```python
from build123d import *

# Parameters (mm, degrees)
SALIENTE_EXTRUIR1_DEPTH             = 30
SALIENTE_EXTRUIR1_2_DEPTH           = 30
SALIENTE_EXTRUIR1_3_DEPTH           = 30
SALIENTE_EXTRUIR1_4_DEPTH           = 30
SALIENTE_EXTRUIR3_REACH             = 48.233
CROQUIS3_W                          = 3.75
CROQUIS3_H                          = 31.257280714
SALIENTE_EXTRUIR3_DIRECTION_2_REACH = 48.233


with BuildPart() as part:
    # Croquis1 → Saliente-Extruir1 (new body)
    with BuildSketch(Plane.XY):
        Polygon((11.559312896, 31.017067239), (16.596862024, 31.017067239), (12.788445042, 0), (7.721401409, -0.240213475), align=None)
    extrude(amount=SALIENTE_EXTRUIR1_DEPTH)



with BuildPart() as body_2:
    # Croquis1 → Saliente-Extruir1 2 (new body)
    with BuildSketch(Plane.XY):
        Polygon((-7.529273594, 31.017067239), (-6.279253351, 20.836469336), (-6.279253351, 4.425451239), (-8.264345654, 20.592730649), (-9.544293245, 31.017067239), align=None)
    extrude(amount=SALIENTE_EXTRUIR1_2_DEPTH)


with BuildPart() as body_3:
    # Croquis1 → Saliente-Extruir1 3 (new body)
    with BuildSketch(Plane.XY):
        Polygon((-11.559312896, 31.017067239), (-7.721401409, -0.240213475), (-12.788445042, 0), (-16.596862024, 31.017067239), align=None)
    extrude(amount=SALIENTE_EXTRUIR1_3_DEPTH)


with BuildPart() as body_4:
    # Croquis1 → Saliente-Extruir1 4 (new body)
    with BuildSketch(Plane.XY):
        Polygon((7.529273594, 31.017067239), (6.279253351, 20.836469336), (6.279253351, 4.425451239), (8.264345654, 20.592730649), (9.544293245, 31.017067239), align=None)
    extrude(amount=SALIENTE_EXTRUIR1_4_DEPTH)


with BuildPart() as part_1:
    add(part.part)

    add(body_2.part)  # Saliente-Extruir3 merges body 2

    add(body_4.part)  # Saliente-Extruir3 merges body 4

    add(body_3.part)  # Saliente-Extruir3 merges body 3
    # Saliente-Extruir3: up to this plane
    saliente_extruir3_end = Plane(origin=(16.596862024, 31.017067239, 30), z_dir=(-0.992546151641322, 0.12186934340514874, 0))
    # Croquis3 → Saliente-Extruir3 (add, up to the surface)
    with BuildSketch(Plane(origin=(0, 0, 0), x_dir=(0, 0, -1), z_dir=(1, 0, 0)), mode=Mode.PRIVATE) as saliente_extruir3_sk1:
        with Locations((-28.125, 15.388426882)):
            Rectangle(CROQUIS3_W, CROQUIS3_H)
    saliente_extruir3_tool1 = split(extrude(saliente_extruir3_sk1.sketch, amount=SALIENTE_EXTRUIR3_REACH, mode=Mode.PRIVATE), bisect_by=saliente_extruir3_end, keep=Keep.BOTH, mode=Mode.PRIVATE)
    add(saliente_extruir3_tool1.solids().sort_by_distance((0, 15.388427, 28.125))[0])
    # Croquis3 → Saliente-Extruir3 (add, up to the surface)
    with BuildSketch(Plane(origin=(0, 0, 0), x_dir=(0, 0, -1), z_dir=(1, 0, 0)), mode=Mode.PRIVATE) as saliente_extruir3_sk2:
        with Locations((-1.875, 15.388426882)):
            Rectangle(CROQUIS3_W, CROQUIS3_H)
    saliente_extruir3_tool2 = split(extrude(saliente_extruir3_sk2.sketch, amount=SALIENTE_EXTRUIR3_REACH, mode=Mode.PRIVATE), bisect_by=saliente_extruir3_end, keep=Keep.BOTH, mode=Mode.PRIVATE)
    add(saliente_extruir3_tool2.solids().sort_by_distance((0, 15.388427, 1.875))[0])

    # Saliente-Extruir3 direction 2: up to this plane
    saliente_extruir3_direction_2_end = Plane(origin=(-16.596862024, 31.017067239, 30), z_dir=(0.992546151641322, 0.12186934340514874, 0))
    # Croquis3 → Saliente-Extruir3 direction 2 (add, up to the surface)
    with BuildSketch(Plane(origin=(0, 0, 0), x_dir=(0, 0, -1), z_dir=(1, 0, 0)), mode=Mode.PRIVATE) as saliente_extruir3_direction_2_sk1:
        with Locations((-28.125, 15.388426882)):
            Rectangle(CROQUIS3_W, CROQUIS3_H)
    saliente_extruir3_direction_2_tool1 = split(extrude(saliente_extruir3_direction_2_sk1.sketch, amount=-SALIENTE_EXTRUIR3_DIRECTION_2_REACH, mode=Mode.PRIVATE), bisect_by=saliente_extruir3_direction_2_end, keep=Keep.BOTH, mode=Mode.PRIVATE)
    add(saliente_extruir3_direction_2_tool1.solids().sort_by_distance((0, 15.388427, 28.125))[0])
    # Croquis3 → Saliente-Extruir3 direction 2 (add, up to the surface)
    with BuildSketch(Plane(origin=(0, 0, 0), x_dir=(0, 0, -1), z_dir=(1, 0, 0)), mode=Mode.PRIVATE) as saliente_extruir3_direction_2_sk2:
        with Locations((-1.875, 15.388426882)):
            Rectangle(CROQUIS3_W, CROQUIS3_H)
    saliente_extruir3_direction_2_tool2 = split(extrude(saliente_extruir3_direction_2_sk2.sketch, amount=-SALIENTE_EXTRUIR3_DIRECTION_2_REACH, mode=Mode.PRIVATE), bisect_by=saliente_extruir3_direction_2_end, keep=Keep.BOTH, mode=Mode.PRIVATE)
    add(saliente_extruir3_direction_2_tool2.solids().sort_by_distance((0, 15.388427, 1.875))[0])


solid = part_1.part
```
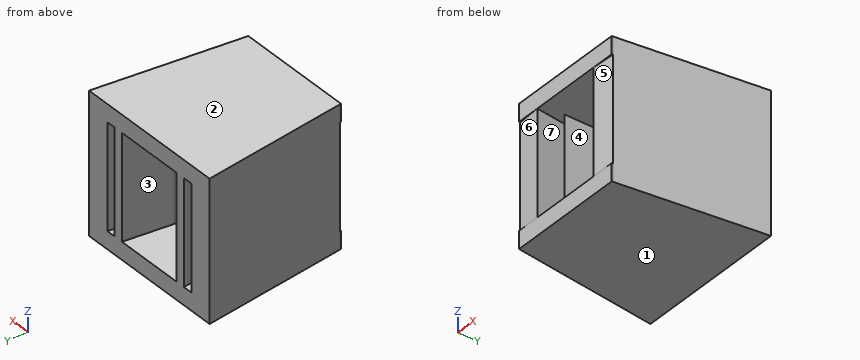
Here's how the part is built. I have some questions about the finished solid (model axes, mm). Face numbers are marked on the shaded views. A direction names the side the tool comes from. Coordinates: 2 decimals unless noted, no trailing zeros. Write each loop counter-clockwise with the first axis right and the second up, starting at its lowest first coordinate (ties: lowest second). Pieces come first, ordered by that corner, then holes. Notation, with made-up numbers: M 23.5,-3.75 L 43.5,-3.75 A19 ccw 43.5,24.25 Z; hole C 78,12 d1. An arc over 180 degrees is marked long. Answer as CSV lines item,"result". Start each with the question number.
Q1. Suppose I cut it at D-D, the plane y = 3. List the corners of the cut face in (x, z) for me.
Q2. Suppose I cut it at B-B, the plane x = -5. List the corners of the cut face in (y, z) for me.
Q3. Will these pins go through, and if not, where does the flat tip stop? pin 1 Ø12 at (y, z) = (13.5, 18.5) entering from +X; pin 2 Ø2 at (y, z) = (18, 15) entering from -X; pin 3 Ø5 at (y, z) = (10.5, 16.5) entering from -X.
Q4. If we mould it in two halves opening along Z, with no side actions, what happens to the marked faces 1, 2 and 3? For each: pulls with the +Z half, pulls with the -Z half, needs draft (parallel to the pull), parting line crosses it, or undercut.
Q5. Suppose I cut it at A-A, the plane z = 24. List the corners of the cut face in (x, y) for me, then the cut area to 3 significant figures.
Q6. Suppose I cut it at C-C, the plane y = 9. List the corners of the cut face in (x, z) for me.
Q7. I need wall thicknesses on probe 1 along X at (y, z) = (29.5, 4); probe 2 along X at (y, z) = (28.5, 7.5); probe 3 along Z at (x, y) = (3, 7). Which ranges of each line are inside material? Lowest first, please. Write a range as [from, to].
Q8. For the marked faces 4, 5, 6 and 7, which set-ups out of +Z, -Z, +X, -X, +Y, -Y let a thin tool reach every point of the face, with its end or its side?
Entries:
1,outline,"M -13.16,0 L 13.16,0 L 13.16,30 L -13.16,30 Z; hole M -8.12,3.75 L 8.12,3.75 L 8.12,26.25 L -8.12,26.25 Z"
2,outline,"M -0.24,0 L 31.02,0 L 31.02,3.75 L -0.24,3.75 Z; M -0.24,26.25 L 31.02,26.25 L 31.02,30 L -0.24,30 Z"
3,pin 1,"stops at x = 15.18"
3,pin 2,"stops at x = -15.12"
3,pin 3,"stops at x = -14.38"
4,face 1,"pulls with the -Z half"
4,face 2,"pulls with the +Z half"
4,face 3,"undercut"
5,outline,"M -16.6,31.02 L -12.79,0 L -7.72,-0.24 L -11.56,31.02 Z; M -9.54,31.02 L -6.28,4.43 L -6.28,20.84 L -7.53,31.02 Z; M 6.28,4.43 L 9.54,31.02 L 7.53,31.02 L 6.28,20.84 Z; M 7.72,-0.24 L 12.79,0 L 16.6,31.02 L 11.56,31.02 Z"
5,area,"388 mm²"
6,outline,"M -13.89,0 L 13.89,0 L 13.89,30 L -13.89,30 Z; hole M -8.86,3.75 L -6.84,3.75 L -6.84,26.25 L -8.86,26.25 Z; hole M -6.28,3.75 L 6.28,3.75 L 6.28,26.25 L -6.28,26.25 Z; hole M 6.84,3.75 L 8.86,3.75 L 8.86,26.25 L 6.84,26.25 Z"
7,probe 1,"x = [-16.41, -11.37], [-9.36, -7.34], [7.34, 9.36], [11.37, 16.41]"
7,probe 2,"x = [-16.29, -11.25], [-9.24, -7.22], [7.22, 9.24], [11.25, 16.29]"
7,probe 3,"z = [0, 3.75], [26.25, 30]"
8,face 4,"+Y, -Y"
8,face 5,"+X, -Y"
8,face 6,"-X, -Y"
8,face 7,"none"
